Could you check a few things on this model? Use its own coordinates, in mm. A direction names the side the tool comes from. Give positions to 0.01 mm unless a question says otherwise; leave off trailing zeros. Order: outer loops, then holes, each group sorted by start corner. A loop starts at its lowest first (then second) coordinate and runs counter-clockwise, first axis right, second up. Notation, with made-up numbers: (33.25, 22.25) -> (50.25, 22.25) arc R9 ccw to (50.25, 31.25) -> close; hole circle Ø1 at (43, -6). An arc over 180 degrees is marked (long way). Answer as CSV lines item,"result". Start each with the question number.
(1) I need wall thicknesses on L1, parallel to Y at x = 36.25, z = -50.8; L2, parallel to Y at x = 38.5, z = -49; L3, parallel to Y at x = 38.5, z = -40.5. Which ranges of each line are inside material? Lowest first, please.
(2) I want a section at B-B (y = 30.5). Please give me the cut outline in (x, z), plus the area to 3 significant figures.
(3) I want a section at A-A (y = 6.35). Please give me the cut outline in (x, z).
(4) We'd pull the mould along Z, two halves only. Please class faces 6 (the face through (38, 38.1, -48)), 7 (the face through (37.51, 6.21, -57.15)), 8 (the face through (36, 26, 38.1)): released by +Z, released by -Z, zero draft, split by the parting line, or undercut.
(5) I want a section at C-C (z = 24). Please give me the cut outline in (x, y).
(6) On a 3-axis mill with a long thin cutter (end or side, diameter ignored), from which of +Z, -Z, +X, -X, +Y, -Y can I reach the whole of each face in a straight line? I mean faces 1 (the face through (36, 26, -38.1)), 2 (the face through (38, 12.7, -48)), 3 (the face through (37.42, 42.9, 40.93)), 4 (the face through (36, 2.54, -1)), 5 (the face through (37, 0, -4)). Say none if no direction works.
(7) Will these pins go through, and if not, where does the flat tip stop? pin 1 Ø3 at (x, y) = (37, 21.5) entering from -Z; pin 2 Ø1.9 at (y, z) = (44.45, 41.275) entering from -X; pin 3 Ø5 at (y, z) = (10, -13.5) entering from -X; pin 4 Ø1.1 at (x, z) = (35.5, -5) entering from +Y.
```python
from build123d import *

# Parameters (mm, degrees)
SKETCH1_W            = 81.28
SKETCH1_H            = 81.28
SKETCH1_W_2          = 76.2
SKETCH1_H_2          = 76.2
BOSS_EXTRUDE1_DEPTH  = 50.8
SKETCH2_W            = 3.81
SKETCH2_H            = 76.2
BOSS_EXTRUDE2_DEPTH  = 2.54
SKETCH3_R            = 1.5748
BOSS_EXTRUDE3_DEPTH  = 6.35
SKETCH4_R            = 1.5875
BOSS_EXTRUDE4_DEPTH  = 6.35
SKETCH6_W            = 74.93
SKETCH6_H            = 50.8
CUT_EXTRUDE1_DEPTH   = 118.45268707
SKETCH7_W            = 2.9972
SKETCH7_H            = 6.35
BOSS_EXTRUDE5_DEPTH  = 1.00076
SKETCH8_W            = 2.9972
SKETCH8_H            = 6.35
BOSS_EXTRUDE6_DEPTH  = 1.99898
BOSS_EXTRUDE6_TAPER  = 3
LPATTERN1_COUNT      = 4
LPATTERN1_PITCH      = 12.7
LPATTERN1_COUNT_DIR2 = 2
LPATTERN1_PITCH_DIR2 = 68.326
SKETCH9_W            = 6.35
SKETCH9_H            = 50.8
BOSS_EXTRUDE7_DEPTH  = 3.81
SKETCH10_R           = 1.5875
CUT_EXTRUDE2_DEPTH   = 77.727341932
SKETCH12_W           = 4.993400043
SKETCH12_H           = 34.528830081
SKETCH12_W_2         = 6.055825583
SKETCH12_H_2         = 9.668072422
SKETCH12_H_3         = 8.28691922
CUT_EXTRUDE3_DEPTH   = 3.81
SKETCH13_W           = 6.35
SKETCH13_H           = 25.4
BOSS_EXTRUDE8_DEPTH  = 3.81
LPATTERN2_COUNT      = 2
LPATTERN2_PITCH      = 82.55


with BuildPart() as part:
    # Sketch1 → Boss-Extrude1 (new body)
    with BuildSketch(Plane(origin=(0, 0, 0), x_dir=(1, 0, 0), z_dir=(0, 1, 0))):
        Rectangle(SKETCH1_W, SKETCH1_H)
        Rectangle(SKETCH1_W_2, SKETCH1_H_2, mode=Mode.SUBTRACT)
    extrude(amount=BOSS_EXTRUDE1_DEPTH)

    # Sketch2 → Boss-Extrude2 (add)
    with BuildSketch(Plane(origin=(0, 0, 0), x_dir=(1, 0, 0), z_dir=(0, 1, 0))):
        with Locations((-36.195, 0)):
            Rectangle(SKETCH2_W, SKETCH2_H)
        with Locations((36.195, 0)):
            Rectangle(SKETCH2_W, SKETCH2_H)
    extrude(amount=BOSS_EXTRUDE2_DEPTH)

    # Sketch3 → Boss-Extrude3 (add)
    with BuildSketch(Plane(origin=(40.64, 0, 0), x_dir=(0, 0, -1), z_dir=(1, 0, 0))):
        with BuildLine():
            Line((50.8, 12.7), (40.64, 12.7))
            Line((40.64, 12.7), (40.64, 0))
            Line((40.64, 0), (50.8, 0))
            ThreePointArc((50.8, 0), (57.15, 6.35), (50.8, 12.7))
        make_face()
        with Locations((50.8, 6.35)):
            Circle(SKETCH3_R, mode=Mode.SUBTRACT)
    boss_extrude3 = extrude(amount=-BOSS_EXTRUDE3_DEPTH)

    # Sketch4 → Boss-Extrude4 (add)
    with BuildSketch(Plane(origin=(40.64, 0, 0), x_dir=(0, 0, -1), z_dir=(1, 0, 0))):
        with BuildLine():
            Line((50.8, 50.8), (40.64, 50.8))
            Line((40.64, 50.8), (40.64, 38.1))
            Line((40.64, 38.1), (50.8, 38.1))
            ThreePointArc((50.8, 38.1), (57.15, 44.45), (50.8, 50.8))
        make_face()
        with Locations((50.8, 44.45)):
            Circle(SKETCH4_R, mode=Mode.SUBTRACT)
    boss_extrude4 = extrude(amount=-BOSS_EXTRUDE4_DEPTH)

    # Mirror1: Boss-Extrude3, Boss-Extrude4 across plane
    add(boss_extrude3.mirror(Plane.ZY))
    add(boss_extrude4.mirror(Plane.ZY))

    # Sketch6 → Cut-Extrude1 (cut, through all)
    with BuildSketch(Plane.XY.offset(40.64)):
        with Locations((-3.175, 25.4)):
            Rectangle(SKETCH6_W, SKETCH6_H)
    extrude(amount=-CUT_EXTRUDE1_DEPTH, mode=Mode.SUBTRACT)

    # Sketch7 → Boss-Extrude5 (add)
    with BuildSketch(Plane.ZY.offset(-38.1)):
        with Locations((-34.16554, 9.017)):
            Rectangle(SKETCH7_W, SKETCH7_H)
    boss_extrude5 = extrude(amount=BOSS_EXTRUDE5_DEPTH)

    # Sketch8 → Boss-Extrude6 (add)
    with BuildSketch(Plane.ZY.offset(-37.09924)):
        with Locations((-34.16554, 9.017)):
            Rectangle(SKETCH8_W, SKETCH8_H)
    boss_extrude6 = extrude(amount=BOSS_EXTRUDE6_DEPTH, taper=BOSS_EXTRUDE6_TAPER)

    # LPattern1: Boss-Extrude5, Boss-Extrude6 4 × 2
    with Locations(*[(0, i * LPATTERN1_PITCH, j * LPATTERN1_PITCH_DIR2) for i in range(LPATTERN1_COUNT) for j in range(LPATTERN1_COUNT_DIR2) if (i, j) != (0, 0)]):
        add(boss_extrude5)
        add(boss_extrude6)

    # Sketch9 → Boss-Extrude7 (add)
    with BuildSketch(Plane(origin=(34.29, 50.8, 40.64), x_dir=(1, 0, 0), z_dir=(0, 0, 1))):
        with Locations((3.175, -25.4)):
            Rectangle(SKETCH9_W, SKETCH9_H)
    extrude(amount=BOSS_EXTRUDE7_DEPTH)

    # Sketch10 → Cut-Extrude2 (cut, through all)
    with BuildSketch(Plane.ZY.offset(-34.29)):
        with Locations((41.275, 44.45)):
            Circle(SKETCH10_R)
        with Locations(Location((41.275, 6.35, 0), (0, 0, 180))):
            Circle(SKETCH10_R)
    cut_extrude2 = extrude(amount=-CUT_EXTRUDE2_DEPTH, mode=Mode.SUBTRACT)

    # Sketch12 → Cut-Extrude3 (cut)
    with BuildSketch(Plane.ZY.offset(-34.29)):
        with Locations((33.961683306, 21.990472175)):
            Rectangle(SKETCH12_W, SKETCH12_H)
        with Locations((-34.13979387, 34.420851005)):
            Rectangle(SKETCH12_W_2, SKETCH12_H_2)
        with Locations((-34.13979387, 8.869516745)):
            Rectangle(SKETCH12_W_2, SKETCH12_H_3)
    extrude(amount=-CUT_EXTRUDE3_DEPTH, mode=Mode.SUBTRACT)

    # Sketch13 → Boss-Extrude8 (add)
    with BuildSketch(Plane(origin=(0, 0, -40.64), x_dir=(-1, 0, 0), z_dir=(0, 0, -1))):
        with Locations((-37.465, 25.4)):
            Rectangle(SKETCH13_W, SKETCH13_H)
    extrude(amount=BOSS_EXTRUDE8_DEPTH)

    # LPattern2: Cut-Extrude2 ×2
    with Locations(*[(0, 0, -i * LPATTERN2_PITCH) for i in range(1, LPATTERN2_COUNT)]):
        add(cut_extrude2, mode=Mode.SUBTRACT)


solid = part.part
```
Final values:
1,L1,"0 to 4.78, 7.92 to 12.7, 38.1 to 42.86, 46.04 to 50.8"
1,L2,"0 to 12.7, 38.1 to 50.8"
1,L3,"0 to 4.96, 7.74 to 43.06, 45.84 to 50.8"
2,outline,"(34.29, -44.45) -> (40.64, -44.45) -> (40.64, 44.45) -> (34.29, 44.45) -> (34.29, 38.1) -> (38.1, 38.1) -> (38.1, -38.1) -> (34.29, -38.1) -> close"
2,area,"274 mm²"
3,outline,"(34.29, -57.15) -> (40.64, -57.15) -> (40.64, -52.37) -> (34.29, -52.37) -> close; (34.29, -49.23) -> (40.64, -49.23) -> (40.64, -42.86) -> (34.29, -42.86) -> close; (34.29, -39.69) -> (40.64, -39.69) -> (40.64, 39.69) -> (34.29, 39.69) -> (34.29, 38.1) -> (38.1, 38.1) -> (38.1, -38.1) -> (34.29, -38.1) -> close; (34.29, 42.86) -> (40.64, 42.86) -> (40.64, 44.45) -> (34.29, 44.45) -> close"
4,face 6,"zero draft"
4,face 7,"released by -Z"
4,face 8,"undercut"
5,outline,"(34.29, 0) -> (40.64, 0) -> (40.64, 50.8) -> (38.1, 50.8) -> (38.1, 2.54) -> (34.29, 2.54) -> close"
6,face 1,"-X, +Y"
6,face 2,"-Z, +X, -X"
6,face 3,"+X, -X"
6,face 4,"-X"
6,face 5,"+Z, -Z, +X, -X, -Y"
7,pin 1,"z = -44.45"
7,pin 2,"through"
7,pin 3,"x = 38.1"
7,pin 4,"y = 2.54"
